Build history of the part. All positions in model axes, mm. A direction names the side the tool comes from. Round coordinates to 2 decimals unless told otherwise and drop trailing zeros. Write each loop counter-clockwise with the first axis right and the second up, starting at its lowest first coordinate (ties: lowest second). Pieces come first, ordered by that corner, then holes.
from build123d import *

# Parameters (mm, degrees)
SKETCH_R        = 48.25
PAD_DEPTH       = 15
SKETCH001_R     = 45.75
POCKET_DEPTH    = 13
SKETCH002_R     = 2
POCKET001_DEPTH = 50
SKETCH003_R     = 20
POCKET002_DEPTH = 2
FILLET_R        = 2
CHAMFER_SIZE    = 1


with BuildPart() as part:
    # Sketch → Pad (new body)
    with BuildSketch(Plane.XY):
        Circle(SKETCH_R)
    extrude(amount=PAD_DEPTH)

    # Sketch001 (on Face2 of Pad) → Pocket (cut)
    with BuildSketch(Plane(origin=(0, 0, 0), x_dir=(1, 0, 0), z_dir=(0, 0, -1))):
        Circle(SKETCH001_R)
    extrude(amount=-POCKET_DEPTH, mode=Mode.SUBTRACT)

    # Sketch002 → Pocket001 (cut, symmetric)
    with BuildSketch(Plane.XZ):
        with Locations((0, 6)):
            Circle(SKETCH002_R)
    extrude(amount=POCKET001_DEPTH, both=True, mode=Mode.SUBTRACT)

    # Sketch003 (on Face3 of Pocket001) → Pocket002 (cut)
    with BuildSketch(Plane.XY.offset(15)):
        Circle(SKETCH003_R)
    extrude(amount=-POCKET002_DEPTH, mode=Mode.SUBTRACT)

    # Fillet
    fillet_edges = [part.edges().sort_by_distance(p)[0] for p in [
        (-48.25, 0, 15),
    ]]
    fillet(fillet_edges, radius=FILLET_R)

    # Chamfer
    chamfer_edges = [part.edges().sort_by_distance(p)[0] for p in [
        (-20, 0, 15),
    ]]
    chamfer(chamfer_edges, length=CHAMFER_SIZE)


solid = part.part
1) Slice it at D-D (z = 11.5). Write the cut outline in (x, y), plus the area to 3 significant figures.
Results:
outline: circle Ø96.5 at (0, 0); hole circle Ø91.5 at (0, 0)
area: 738 mm2
2) Mould opens along Z. For faces 1 (the cylindrical face through (-4.336, -19.524, 13.507)), 2 (the cylindrical face through (0, -47, 8)), 3 (the flat face through (18, -43, 0)) say: released by +Z, released by -Z, zero draft, split by the parting line, or undercut.
Results:
face 1: zero draft
face 2: undercut
face 3: released by -Z
3) Slice it at A-A (x = 0). Write the cut outline in (y, z), plus the area to 3 significant figures.
Results:
outline: (-48.25, 0) - (-45.75, 0) - (-45.75, 4) - (-48.25, 4) - close; (-48.25, 8) - (-45.75, 8) - (-45.75, 13) - (-20, 13) - (-20, 14) - (-21, 15) - (-46.25, 15) arc R2 ccw to (-48.25, 13) - close; (20, 13) - (45.75, 13) - (45.75, 8) - (48.25, 8) - (48.25, 13) arc R2 ccw to (46.25, 15) - (21, 15) - (20, 14) - close; (45.75, 0) - (48.25, 0) - (48.25, 4) - (45.75, 4) - close
area: 155 mm2
4) Pin check, flat tips, straight feed: pin 1 Ø4 at (x, y) = (6, 17.5) entering from -Z; pin 2 Ø1 at (x, z) = (13.5, 6) entering from -Y; pin 3 Ø1 at (y, z) = (29, 6) entering from +X. Stop position of each tip, or through.
Results:
pin 1: stops at z = 13
pin 2: stops at y = -46.47
pin 3: stops at x = 38.93
5) Slice it at B-B (y = 0). Write the cut outline in (x, z), plus the area to 3 significant figures.
Results:
outline: (-48.25, 0) - (-45.75, 0) - (-45.75, 13) - (-20, 13) - (-20, 14) - (-21, 15) - (-46.25, 15) arc R2 ccw to (-48.25, 13) - close; (20, 13) - (45.75, 13) - (45.75, 0) - (48.25, 0) - (48.25, 13) arc R2 ccw to (46.25, 15) - (21, 15) - (20, 14) - close
area: 175 mm2
6) Wall check: L1, parallel to Z at x = 0, y = 46.4; L2, parallel to Z at x = 11.5, y = 26.5; L3, parallel to Y at x = -25.5, z = 4.5. Give the ranges that are in metal, low to high.
Results:
L1: z = 0 to 4, 8 to 14.99
L2: z = 13 to 15
L3: y = -40.96 to -37.98, 37.98 to 40.96
7) Which spindle directions (+Z, -Z, +X, -X, +Y, -Y) get a long thin tool onto all of the face, cutting with end or side? Do faces 4 (the cylindrical face through (-48.203, 2.121, 6.409)), 5 (the cylindrical face through (43.64, -13.74, 6.41)). Say none if no direction does.
Results:
face 4: +Z, -Z
face 5: -Z
